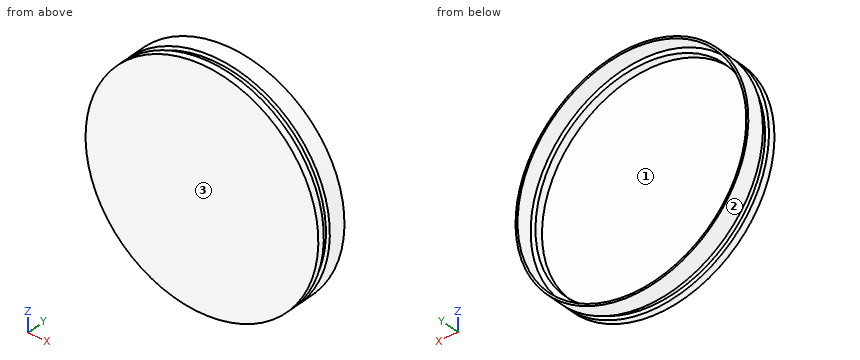
from build123d import *

# Parameters (mm, degrees)
SKETCH_1_R       = 72.25
SKETCH_1_R_2     = 71
EXTRUDE_1_DEPTH  = 20
SKETCH_1_6_R     = 71
SKETCH_1_6_R_2   = 68
EXTRUDE_3_DEPTH  = 10
SKETCH_2_W       = 2
SKETCH_2_H       = 3
CHAMFER_1_SIZE   = 3
CHAMFER_1_SIZE_2 = 0.803847577
CHAMFER_2_SIZE   = 0.803847577
CHAMFER_2_SIZE_2 = 3
SKETCH_1_8_R     = 68
SKETCH_1_8_R_2   = 62.25
EXTRUDE_5_DEPTH  = 5


with BuildPart() as part:
    # 草圖1 → 填料-伸長1 (new body)
    with BuildSketch(Plane(origin=(0, 0, 0), x_dir=(1, 0, 0), z_dir=(0, 1, 0))):
        with Locations(Location((0, 0, 0), (0, 0, 270))):
            Circle(SKETCH_1_R)
        with Locations(Location((0, 0, 0), (0, 0, 270))):
            Circle(SKETCH_1_R_2, mode=Mode.SUBTRACT)
    extrude(amount=EXTRUDE_1_DEPTH)

    # 草圖1<6> → 填料-伸長3 (add)
    with BuildSketch(Plane(origin=(0, 0, 0), x_dir=(1, 0, 0), z_dir=(0, 1, 0))):
        with Locations(Location((0, 0, 0), (0, 0, 270))):
            Circle(SKETCH_1_6_R)
        with Locations(Location((0, 0, 0), (0, 0, 270))):
            Circle(SKETCH_1_6_R_2, mode=Mode.SUBTRACT)
    extrude(amount=EXTRUDE_3_DEPTH)

    # 草圖2 → 除料-旋轉1 (revolve, cut)
    with BuildSketch(Plane.XY, mode=Mode.PRIVATE) as cut_revolve_1_sk:
        with Locations((71.25, 6.5)):
            Rectangle(SKETCH_2_W, SKETCH_2_H)
    revolve(cut_revolve_1_sk.sketch.rotate(Axis((0, 0, 0), (0, 1, 0)), 90), axis=Axis((0, 0, 0), (0, 1, 0)), mode=Mode.SUBTRACT)

    # 導角1
    # the kernel refuses this chamfer: 3, 0.803847577 mm, written as the material it takes off along each edge
    with BuildSketch(Plane(origin=(0, 8, 0), x_dir=(0, 0, 1), z_dir=(1, 0, 0))) as chamfer_1_piece_1_section:
        Polygon((72.25 - CHAMFER_1_SIZE, 0), (72.25, -CHAMFER_1_SIZE_2), (72.25, 0), align=None)
    chamfer_1_piece_1 = revolve(axis=Axis((0, 8, 0), (0, -1, 0)), mode=Mode.PRIVATE)
    chamfer_1_piece_1 = chamfer_1_piece_1 - Plane(origin=(0, 8.471650201, 0), x_dir=(0, 0, -1), z_dir=(0, 1, 0)) * Cylinder(70.25, 289, mode=Mode.PRIVATE)
    add(chamfer_1_piece_1, mode=Mode.SUBTRACT)

    # 導角2
    # the kernel refuses this chamfer: 3, 0.803847577 mm, written as the material it takes off along each edge
    with BuildSketch(Plane(origin=(0, 5, 0), x_dir=(0, 0, 1), z_dir=(1, 0, 0))) as chamfer_2_piece_1_section:
        Polygon((72.25, CHAMFER_2_SIZE), (72.25 - CHAMFER_2_SIZE_2, 0), (72.25, 0), align=None)
    chamfer_2_piece_1 = revolve(axis=Axis((0, 5, 0), (0, -1, 0)), mode=Mode.PRIVATE)
    chamfer_2_piece_1 = chamfer_2_piece_1 - Plane(origin=(0, 4.528349799, 0), x_dir=(0, 0, -1), z_dir=(0, 1, 0)) * Cylinder(70.25, 289, mode=Mode.PRIVATE)
    add(chamfer_2_piece_1, mode=Mode.SUBTRACT)

    # 草圖1<8> → 填料-伸長5 (add)
    # profile 1 of 2: a face of its own
    with BuildSketch(Plane(origin=(0, 0, 0), x_dir=(1, 0, 0), z_dir=(0, 1, 0))):
        with Locations(Location((0, 0, 0), (0, 0, 270))):
            Circle(SKETCH_1_8_R)
        Circle(SKETCH_1_8_R_2, mode=Mode.SUBTRACT)
    # profile 2 of 2: a face of its own
    with BuildSketch(Plane(origin=(0, 0, 0), x_dir=(1, 0, 0), z_dir=(0, 1, 0))):
        Circle(SKETCH_1_8_R_2)
    extrude(amount=EXTRUDE_5_DEPTH)


solid = part.part
The model under review builds one solid part; all positions refer to its coordinate system, in mm. Face numbers are marked on the shaded views. Round coordinates to 2 decimals unless told otherwise and drop trailing zeros. Order: outer loops, then holes, each group sorted by start corner. A loop starts at its lowest first (then second) coordinate and runs counter-clockwise, first axis right, second up. Notation, with made-up numbers: (-1.5, 61) -> (54.5, 61) arc R18 ccw to (54.5, 75) -> close; hole circle Ø6 at (25.5, -35.5). An arc over 180 degrees is marked (long way). Use CSV: the item, a comma, the result in double quotes. Start each with the question number.
(1) Consider section B-B on z = 0. Write out the cut boundary in (x, y).
(2) Consider section C-C on y = 2.5. Write out the cut boundary in (x, z).
(3) Consider section A-A on x = 0. Write out the cut boundary in (y, z), and give its area (3 significant figures).
(4) Wall thickness on probe 1 along X at (y, z) = (15.75, 0); probe 2 along X at (y, z) = (7.7, 0); probe 3 along Y at (x, z) = (-24.5, -11): over which ranges is each line inside the solid? List them lowest first. Write a range as from..to.
(5) Mouldability with a two-part tool opening along Z and no side actions: class the marked faces 1, 2 and 3 as pulls with the +Z half, pulls with the -Z half, needs draft (parallel to the pull), parting line crosses it, or undercut.
(6) Insertion check: pin 1 (5 mm diameter, centred on x = -14, y = 10, fed in from -Z); pin 2 (2 mm diameter, centred on x = -30.5, y = 2, fed in from +Z); pin 3 (8 mm diameter, centred on y = 3.5, z = -34, fed in from -X). Each pin has a flat end and moves straight along its axis. Give the tip position at first contact, or say it passes through.
Responses:
1,outline,"(-72.25, 0) -> (72.25, 0) -> (72.25, 4.2) -> (70.25, 4.73) -> (70.25, 8.27) -> (72.25, 8.8) -> (72.25, 20) -> (71, 20) -> (71, 10) -> (68, 10) -> (68, 5) -> (-68, 5) -> (-68, 10) -> (-71, 10) -> (-71, 20) -> (-72.25, 20) -> (-72.25, 8.8) -> (-70.25, 8.27) -> (-70.25, 4.73) -> (-72.25, 4.2) -> close"
2,outline,"circle Ø144.5 at (0, 0)"
3,outline,"(0, -72.25) -> (4.2, -72.25) -> (4.73, -70.25) -> (8.27, -70.25) -> (8.8, -72.25) -> (20, -72.25) -> (20, -71) -> (10, -71) -> (10, -68) -> (5, -68) -> (5, 68) -> (10, 68) -> (10, 71) -> (20, 71) -> (20, 72.25) -> (8.8, 72.25) -> (8.27, 70.25) -> (4.73, 70.25) -> (4.2, 72.25) -> (0, 72.25) -> close"
3,area,"774 mm²"
4,probe 1,"-72.25..-71, 71..72.25"
4,probe 2,"-70.25..-68, 68..70.25"
4,probe 3,"0..5"
5,face 1,"undercut"
5,face 2,"parting line crosses it"
5,face 3,"needs draft"
6,pin 1,"z = -71.33"
6,pin 2,"z = 65.95"
6,pin 3,"x = -65.73"
